Source: CAD feature listing. Evaluate the final solid. Frame: model axes, mm. Face numbers are marked on the shaded views. A direction names the side the tool comes from. Round coordinates to 2 decimals unless told otherwise and drop trailing zeros. Order: outer loops, then holes, each group sorted by start corner. A loop starts at its lowest first (then second) coordinate and runs counter-clockwise, first axis right, second up. Notation, with made-up numbers: (-33.75, 31) -> (7.25, 31) arc R8 ccw to (7.25, 43) -> close; hole circle Ø11 at (-14, 19.5). An arc over 180 degrees is marked (long way). Write item = value, one per line. Start each with the question number.
(1) Cut plane A-A on x = 13. Return the cut outline in (y, z), then the cut area to 3 significant figures.
(2) Cut plane B-B on y = 0.75. Return the cut outline in (x, z), then the cut area to 3 significant figures.
(3) Contact query for flat-ended pins moving along their axis: pin 1 Ø0.8 at (x, y) = (-3.5, -5.5) entering from +Z; pin 2 Ø1.6 at (y, z) = (-5.5, 1.5) entering from +X; pin 3 Ø3 at (y, z) = (-6, 1) entering from -X. Output: stop coordinate, or through.
(4) Cut plane C-C on z = -8. Return the cut outline in (x, y), then the cut area to 3 significant figures.
(5) Cut plane D-D on y = -5. Return the cut outline in (x, z).
(6) Reachability of the marked faces 1, 2 and 3 from +Z, -Z, +X, -X, +Y, -Y: full face, straight path, thin tool, end or side. Return the list, or none.
(7) Ray query, line 1 (X direction, y = 3.25, z = -2); line 2 (Y direction, x = 1.5, z = 1); line 3 (Y direction, x = -13.75, z = 2). Return the intervals inside material, ascending.
from build123d import *

# Parameters (mm, degrees)
F1_DEPTH = 10
F2_W     = 2.4
F2_H     = 12.2
F2_W_2   = 3.2
F2_H_2   = 1.8
F3_DEPTH = 2.7
F4_W     = 3.2
F4_H     = 12.2
F5_DEPTH = 0.5
F6_DEPTH = 3
F7_SIZE2 = 3.2
F7_SIZE  = 4
F8_R     = 5


with BuildPart() as f1:
    # F0 (on Top) → F1 (new body, symmetric)
    with BuildSketch(Plane.XY):
        Polygon((-9.25, -1.25), (-13.75, -1.25), (-18.25, -1.25), (-18.25, -4.25), (0, -4.25), (18.25, -4.25), (18.25, -1.25), (13.75, -1.25), (9.25, -1.25), (0, -1.25), align=None)
        Polygon((9.25, 4.5), (9.25, -1.25), (13.75, -1.25), (18.25, -1.25), (18.25, 4.5), align=None)
        with BuildLine():
            ThreePointArc((15, 0), (14.6338834765, -0.8838834765), (13.75, -1.25))
            ThreePointArc((13.75, -1.25), (12.8661165235, 0.8838834765), (15, 0))
        make_face(mode=Mode.SUBTRACT)
        Polygon((-18.25, -1.25), (-13.75, -1.25), (-9.25, -1.25), (-9.25, 4.5), (-18.25, 4.5), align=None)
        with BuildLine():
            ThreePointArc((-13.75, -1.25), (-14.6338834765, 0.8838834765), (-12.5, 0))
            ThreePointArc((-12.5, 0), (-12.8661165235, -0.8838834765), (-13.75, -1.25))
        make_face(mode=Mode.SUBTRACT)
    extrude(amount=F1_DEPTH, both=True)

    # F2 (on face) → F3 (join)
    with BuildSketch(Plane.XZ.offset(4.25)):
        with Locations((0, 0.9)):
            Rectangle(F2_W, F2_H)
        with Locations((-2.8, -6.1)):
            Rectangle(F2_W_2, F2_H_2)
        with Locations((0, -6.1)):
            Rectangle(F2_W, F2_H_2)
        with Locations((2.8, -6.1)):
            Rectangle(F2_W_2, F2_H_2)
    extrude(amount=F3_DEPTH)

    # F4 (on face) → F5 (join)
    with BuildSketch(Plane.XZ.offset(6.95)):
        with Locations((2.8, 0.9)):
            Rectangle(F4_W, F4_H)
        Polygon((-4.4, -5.2), (-4.4, -7), (4.4, -7), (4.4, -5.2), (1.2, -5.2), (1.2, 7), (-1.2, 7), (-1.2, -5.2), align=None)
        with Locations((-2.8, 0.9)):
            Rectangle(F4_W, F4_H)
    extrude(amount=F5_DEPTH)

    # F6 (add, through all): a face of the model
    f6_faces = [f1.faces().sort_by_distance(p)[0] for p in [
        (0, -5.85, -7),
    ]]
    extrude(f6_faces, amount=F6_DEPTH)

    # F7
    f7_edges = [f1.edges().sort_by_distance(p)[0] for p in [
        (0, -7.45, -10),
    ]]
    f7_side = f1.faces().sort_by_distance((0, -7.45, -1.5))[0]
    chamfer(f7_edges, length=F7_SIZE, length2=F7_SIZE2, reference=f7_side)

    # F8
    f8_edges = [f1.edges().sort_by_distance(p)[0] for p in [
        (0, -7.45, -6),
    ]]
    fillet(f8_edges, radius=F8_R)


solid = f1.part
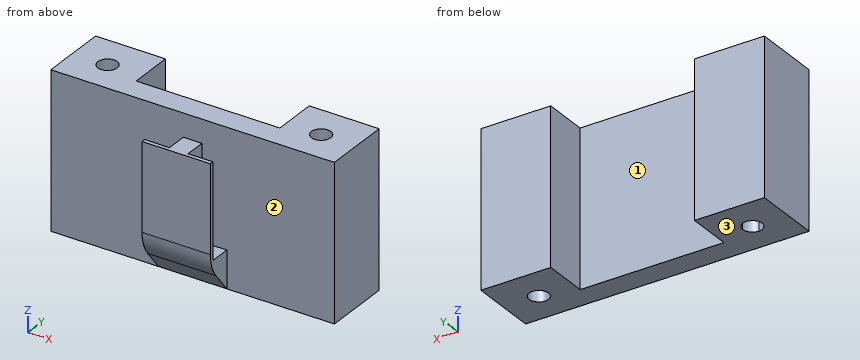
Evaluation:
q1.outline = (-4.25, -10) -> (-1, -10) -> (-1, 10) -> (-4.25, 10) -> close; (1, -10) -> (4.5, -10) -> (4.5, 10) -> (1, 10) -> close
q1.area = 135 mm^2
q2.outline = (-18.25, -10) -> (-14.75, -10) -> (-14.75, 10) -> (-18.25, 10) -> close; (-12.75, -10) -> (-9.25, -10) -> (-9.25, 10) -> (-12.75, 10) -> close; (9.25, -10) -> (12.75, -10) -> (12.75, 10) -> (9.25, 10) -> close; (14.75, -10) -> (18.25, -10) -> (18.25, 10) -> (14.75, 10) -> close
q2.area = 280 mm^2
q3.pin_1 = -5.2
q3.pin_2 = 1.2
q3.pin_3 = -4.4
q4.outline = (-18.25, -4.25) -> (-4.4, -4.25) -> (-4.4, -5.85) -> (4.4, -5.85) -> (4.4, -4.25) -> (18.25, -4.25) -> (18.25, 4.5) -> (9.25, 4.5) -> (9.25, -1.25) -> (-9.25, -1.25) -> (-9.25, 4.5) -> (-18.25, 4.5) -> close; hole circle Ø2.5 at (-13.75, 0); hole circle Ø2.5 at (13.75, 0)
q4.area = 217 mm^2
q5.outline = (-4.4, -9.06) -> (4.4, -9.06) -> (4.4, -5.2) -> (1.2, -5.2) -> (1.2, 7) -> (-1.2, 7) -> (-1.2, -5.2) -> (-4.4, -5.2) -> close
q6.face_1 = +Z, -Z, +Y
q6.face_2 = +Z
q6.face_3 = -Z, +X, -X, +Y, -Y
q7.line_1 = -18.25 to -9.25, 9.25 to 18.25
q7.line_2 = -7.45 to -6.95, -4.25 to -1.25
q7.line_3 = -4.25 to -1.25, 1.25 to 4.5
